Model file for the job. Use its own axes, mm. A direction names the side the tool comes from. Round coordinates to 2 decimals unless told otherwise and drop trailing zeros. Order: outer loops, then holes, each group sorted by start corner. A loop starts at its lowest first (then second) coordinate and runs counter-clockwise, first axis right, second up. Notation, with made-up numbers: M -39.75,89.25 L 16.25,89.25 A26 cw 16.25,111.25 Z; hole C 19.5,-0.75 d11. An arc over 180 degrees is marked long. Return JSON: item names as keys, results as strings. Group by question number.
Item 1: Slice it at B-B on z = -11.5. Write the cut outline in (x, y), then the cut area to 3 significant figures.
Item 2: Slice it at C-C on x = 24. Write the cut outline in (y, z).
Item 3: Which spindle directions (+Z, -Z, +X, -X, +Y, -Y) get a long thin tool onto all of the face, cutting with end or side? Do faces 4 (the face through (2.056, 10.07, -2.681)), 5 (the face through (-34.265, -14.79, 7.609)). Say none if no direction does.
Item 4: Slice it at D-D on y = 1.5. Write the cut outline in (x, z).
Item 5: Probe line 1 along Z through (x, y) = (0, 7); line 2 along Y through (x, z) = (-10, -32.5). List the from-to ranges inside material, lowest first.
Item 6: Pull direction Z, two halves, no side cores. Call faces 1 (the face through (0, 0, 0)), 2 (the face through (-35.4, -30, 0.2)), 3 (the face through (39.913, -7.185, -2.637)): pulls with the +Z half, pulls with the -Z half, needs draft (parallel to the pull), parting line crosses it, or undercut.
Item 7: Slice it at A-A on y = -26. Write the cut outline in (x, z), then the cut area to 3 significant figures.
Item 8: Pin check, flat tips, straight feed: pin 1 Ø21 at (x, z) = (-16, -6.5) entering from -Y; pin 2 Ø1.5 at (y, z) = (4, -24.5) entering from -X; pin 3 Ø2 at (x, z) = (28.5, -28.5) entering from +Y; pin 4 Ø3 at (x, y) = (8.5, 2.5) entering from -Z. Stop position of each tip, or through.
from build123d import *

# Parameters (mm, degrees)
ESQUISSE1_R           = 40
BOSS_EXTRU_1_DEPTH    = 15
ESQUISSE5_R           = 40
ESQUISSE5_R_2         = 35.1
BOSS_EXTRU_2_DEPTH    = 30
D_GAGEMENT_M41_REACH  = 97.28
D_GAGEMENT_M41_BORE_R = 2.25


with BuildPart() as part:
    # Esquisse1 → Boss.-Extru.1 (new body)
    with BuildSketch(Plane(origin=(0, 0, 0), x_dir=(1, 0, 0), z_dir=(0, 1, 0))):
        with Locations(Location((0, 0, 0), (0, 0, 270))):
            Circle(ESQUISSE1_R)
    extrude(amount=BOSS_EXTRU_1_DEPTH)

    # Esquisse5 → Boss.-Extru.2 (add)
    with BuildSketch(Plane.XZ):
        with Locations(Location((0, 0, 0), (0, 0, 270))):
            Circle(ESQUISSE5_R)
        with Locations(Location((0, 0, 0), (0, 0, 270))):
            Circle(ESQUISSE5_R_2, mode=Mode.SUBTRACT)
    extrude(amount=BOSS_EXTRU_2_DEPTH)

    # Dégagement M41 bore (on position points) → Dégagement M41 (cut, up to next)
    with BuildSketch(Plane(origin=(39.999952301, -17.76077449, -0.061772988), x_dir=(0.0015443247, 0, 0.99999880753), z_dir=(0.99999880753, 0, -0.0015443247)), mode=Mode.PRIVATE) as d_gagement_m41_sk1:
        Circle(D_GAGEMENT_M41_BORE_R)
    d_gagement_m41_tool1 = extrude(d_gagement_m41_sk1.sketch, amount=-D_GAGEMENT_M41_REACH, mode=Mode.PRIVATE) & part.part
    add(d_gagement_m41_tool1.solids().sort_by_distance((39.999952, -17.760774, -0.061773))[0], mode=Mode.SUBTRACT)

    # Esquisse11 → Dégagement 1/41 (revolve, cut)
    with BuildSketch(Plane(origin=(0, 15, 0), x_dir=(0, 0, 1), z_dir=(1, 0, 0))):
        Polygon((0, 0), (0, 12.029827343), (3.3782, 10), (3.3782, 0), align=None)
    revolve(axis=Axis((0, 21.35, 0), (0, -1, 0)), mode=Mode.SUBTRACT)


solid = part.part
Output values:
{
 "1": {"outline": "M -38.31,-30 L -33.16,-30 L -33.16,0 L 33.16,0 L 33.16,-30 L 38.31,-30 L 38.31,15 L -38.31,15 Z", "area": "1,460 mm²"},
 "2": {"outline": "M -30,-32 L 15,-32 L 15,32 L -30,32 L -30,25.61 L 0,25.61 L 0,-25.61 L -30,-25.61 Z"},
 "3": {"face 4": "+Y", "face 5": "-Y"},
 "4": {"outline": "C 0,0 d80"},
 "5": {"line 1": "-40 to -3.38, 3.38 to 40", "line 2": "0 to 15"},
 "6": {"face 1": "undercut", "face 2": "needs draft", "face 3": "parting line crosses it"},
 "7": {"outline": "C 0,0 d80; hole C 0,0 d70.2", "area": "1,160 mm²"},
 "8": {"pin 1": "y = 0", "pin 2": "x = -32.19", "pin 3": "y = 15", "pin 4": "z = -39.38"}
}
